Print and shaded views of the part. All mm, measured from the part's lowest x, y and z. Give positions to 0.01 mm unless a question says otherwise; leave off trailing zeros. Loops run counter-clockwise (first coordinate to the right, second up) from the corner with the lowest first, then second, coordinate; pieces in that order, holes last. Notation, with made-up numbers: M 4.25,24 L 35.25,24 A14 cw 35.25,40 Z; hole C -37.75,35 d11. An arc over 180 degrees is marked long. Answer as CSV lines item,"result".
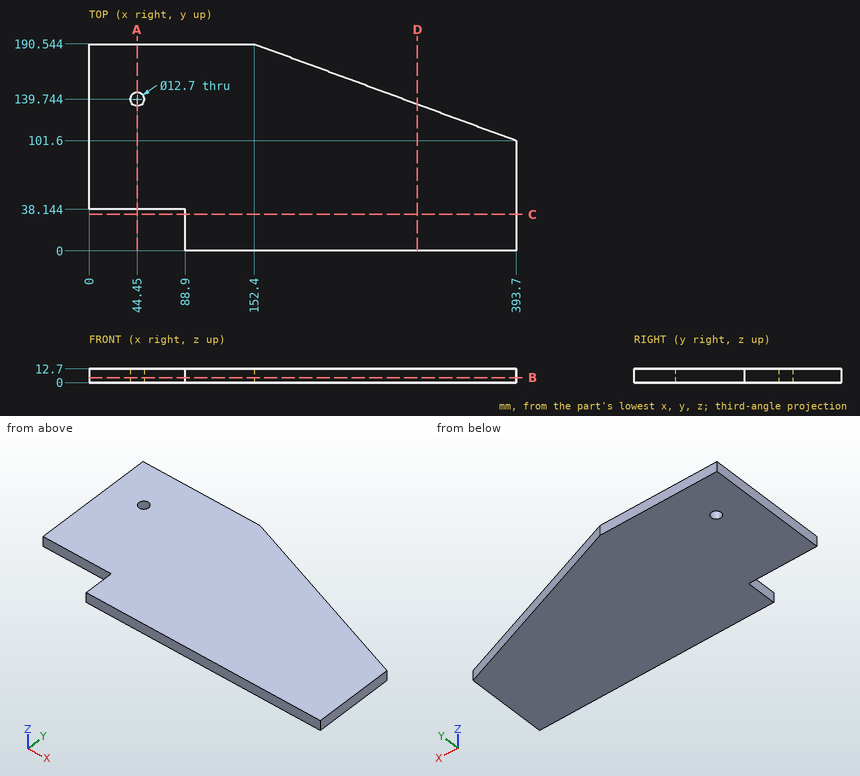
Q1. Wall check: line 1 (Y direction, x = 44.45, z = 7.5); line 2 (X direction, y = 8, z = 5); line 3 (Y direction, x = 37.5, z = 4.25). Give the ranges that are in metal, low to high. Write a range as [from, to].
Solution:
line 1,"y = [38.14, 133.39], [146.09, 190.54]"
line 2,"x = [88.9, 393.7]"
line 3,"y = [38.14, 190.54]"
Q2. Cut at D-D (x = 302.5). Write the cut outline in (y, z), and give its area (3 significant figures).
Solution:
outline,"M 0,0 L 135.22,0 L 135.22,12.7 L 0,12.7 Z"
area,"1,720 mm²"
Q3. Pin check, flat tips, straight feed: P1, Ø6.5, axis at x = 25, z = 5.5, coming from the -Y side; P2, Ø2, axis at x = 353.5, z = 4, coming from the +Y side. Stop position of each tip, or through.
Solution:
P1,"stops at y = 38.14"
P2,"stops at y = 116.79"
Q4. Cut at B-B (z = 4.5). Write the cut outline in (x, y), and give its area (3 significant figures).
Solution:
outline,"M 0,38.14 L 88.9,38.14 L 88.9,0 L 393.7,0 L 393.7,101.6 L 152.4,190.54 L 0,190.54 Z; hole C 44.45,139.74 d12.7"
area,"60,800 mm²"
Q5. Cut at A-A (x = 44.45). Write the cut outline in (y, z).
Solution:
outline,"M 38.14,0 L 133.39,0 L 133.39,12.7 L 38.14,12.7 Z; M 146.09,0 L 190.54,0 L 190.54,12.7 L 146.09,12.7 Z"
Q6. Cut at C-C (y = 33.5). Write the cut outline in (x, z), and give its area (3 significant figures).
Solution:
outline,"M 88.9,0 L 393.7,0 L 393.7,12.7 L 88.9,12.7 Z"
area,"3,870 mm²"
